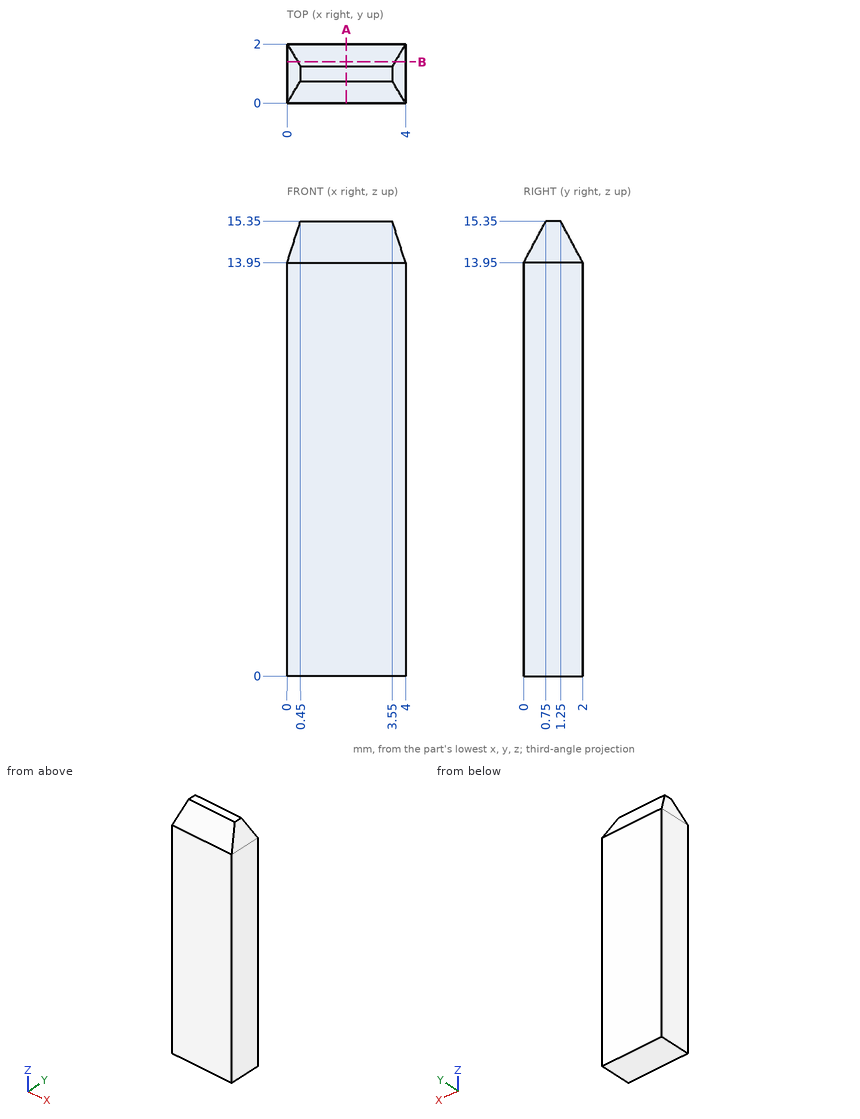
Check sheet for the drawn part. Datum: minimum x, y, z corner. Units: mm. Round coordinates to 2 decimals unless told otherwise and drop trailing zeros. Loops run counter-clockwise (first coordinate to the right, second up) from the corner with the lowest first, then second, coordinate; pieces in that order, holes last. Notation, with made-up numbers: (-40, -16) - (14, -16) arc R27 cw to (14, 6) - close; hole circle Ø6 at (64.25, 66.25). An arc over 180 degrees is marked (long way). Use one line per item in the form item = value.
1. Scan lines: probe 1 along Y at (x, z) = (1.55, 14.25); probe 2 along Z at (x, y) = (1.6, 1.6); probe 3 along Z at (x, y) = (0.7, 0.65). Record each from-to range of solid material in increasing order.
A:
probe_1 = 0.16 to 1.84
probe_2 = 0 to 14.7
probe_3 = 0 to 15.16
2. Section check A-A on x = 2. Record the cut outline in (y, z).
A:
outline = (0, 0) - (2, 0) - (2, 13.95) - (1.25, 15.35) - (0.75, 15.35) - (0, 13.95) - close
3. Section check B-B on y = 1.4. Record the cut outline in (x, z), and give its area (3 significant figures).
A:
outline = (0, 0) - (4, 0) - (4, 13.95) - (3.64, 15.07) - (0.36, 15.07) - (0, 13.95) - close
area = 59.9 mm²
